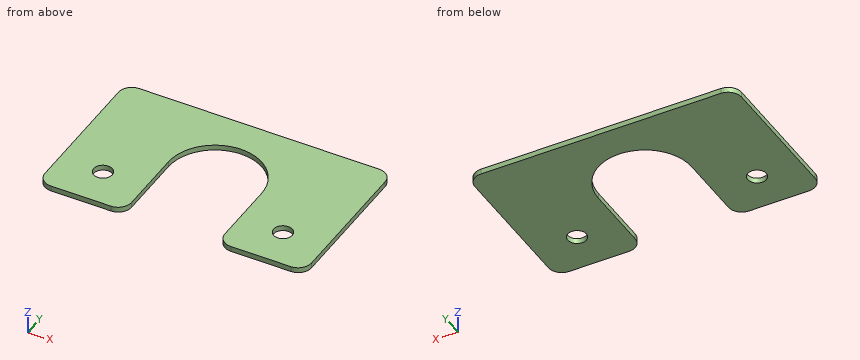
```python
from build123d import *

# Parameters (mm, degrees)
SKETCH1_W          = 100
SKETCH1_H          = 60
BASE_FLANGE1_DEPTH = 2
CUT_EXTRUDE1_DEPTH = 10
FILLET1_R          = 5
SKETCH7_R          = 3.5
CUT_EXTRUDE2_DEPTH = 10
FILLET2_R          = 5


# Sheet-metal steps are written as plain solids
with BuildPart() as part:
    # Sketch1 → Base-Flange1 (new body)
    with BuildSketch(Plane.XY):
        Rectangle(SKETCH1_W, SKETCH1_H)
    extrude(amount=-BASE_FLANGE1_DEPTH)

    # Sketch6 → Cut-Extrude1 (cut)
    with BuildSketch(Plane.XY):
        with BuildLine():
            Line((-17.5, 0), (-17.5, -30))
            Line((-17.5, -30), (17.5, -30))
            Line((17.5, -30), (17.5, 0))
            ThreePointArc((17.5, 0), (0, 17.5), (-17.5, 0))
        make_face()
    extrude(amount=-CUT_EXTRUDE1_DEPTH, mode=Mode.SUBTRACT)

    # Fillet1
    fillet1_edges = [part.edges().sort_by_distance(p)[0] for p in [
        (17.5, -30, -1),
        (50, -30, -1),
        (-50, -30, -1),
        (-50, 30, -1),
        (50, 30, -1),
    ]]
    fillet(fillet1_edges, radius=FILLET1_R)

    # Sketch7 → Cut-Extrude2 (cut)
    with BuildSketch(Plane.XY):
        with Locations((-33.75, -15)):
            Circle(SKETCH7_R)
        with Locations((33.75, -15)):
            Circle(SKETCH7_R)
    extrude(amount=-CUT_EXTRUDE2_DEPTH, mode=Mode.SUBTRACT)

    # Fillet2
    fillet2_edges = [part.edges().sort_by_distance(p)[0] for p in [
        (-17.5, -30, -1),
    ]]
    fillet(fillet2_edges, radius=FILLET2_R)


solid = part.part
```
Could you check a few things on this model? Use its own coordinates, in mm. Round coordinates to 2 decimals unless told otherwise and drop trailing zeros. Loops run counter-clockwise (first coordinate to the right, second up) from the corner with the lowest first, then second, coordinate; pieces in that order, holes last. Notation, with made-up numbers: (-30, 37) - (-26, 37) arc R22 ccw to (-26, 70) - close; hole circle Ø8 at (60, -7). An arc over 180 degrees is marked (long way). Use CSV: the item, a comma, the result in double quotes.
Item 1: If we section it at A-A on x = -33.75: List the corners of the cut face in (y, z) for me.
Here are the results:
outline,"(-30, -2) - (-18.5, -2) - (-18.5, 0) - (-30, 0) - close; (-11.5, -2) - (30, -2) - (30, 0) - (-11.5, 0) - close"
Item 2: I need wall thicknesses on L1, parallel to X at y = -19.5, z = -1.55; L2, parallel to Y at x = 33.75, z = -0.7; L3, parallel to X at y = 13, z = -1.3. Which ranges of each line are inside material? Lowest first, please. Write a range as [from, to].
Here are the results:
L1,"x = [-50, -17.5], [17.5, 50]"
L2,"y = [-30, -18.5], [-11.5, 30]"
L3,"x = [-50, -11.72], [11.72, 50]"
Item 3: If we section it at D-D on y = -15: List the corners of the cut face in (x, z) for me, then the cut area to 3 significant figures.
Here are the results:
outline,"(-50, -2) - (-37.25, -2) - (-37.25, 0) - (-50, 0) - close; (-30.25, -2) - (-17.5, -2) - (-17.5, 0) - (-30.25, 0) - close; (17.5, -2) - (30.25, -2) - (30.25, 0) - (17.5, 0) - close; (37.25, -2) - (50, -2) - (50, 0) - (37.25, 0) - close"
area,"102 mm²"
Item 4: If we section it at C-C on z = -1.1: List the corners of the cut face in (x, y) for me, then the cut area to 3 significant figures.
Here are the results:
outline,"(-50, -25) arc R5 ccw to (-45, -30) - (-22.5, -30) arc R5 ccw to (-17.5, -25) - (-17.5, 0) arc R17.5 cw to (17.5, 0) - (17.5, -25) arc R5 ccw to (22.5, -30) - (45, -30) arc R5 ccw to (50, -25) - (50, 25) arc R5 ccw to (45, 30) - (-45, 30) arc R5 ccw to (-50, 25) - close; hole circle Ø7 at (-33.75, -15); hole circle Ø7 at (33.75, -15)"
area,"4,360 mm²"
Item 5: If we section it at B-B on y = -24: List the corners of the cut face in (x, z) for me.
Here are the results:
outline,"(-50, -2) - (-17.5, -2) - (-17.5, 0) - (-50, 0) - close; (17.5, -2) - (50, -2) - (50, 0) - (17.5, 0) - close"
